Design review of the part built by this model. Coordinates are the model's own, in mm. A direction names the side the tool comes from. Give positions to 0.01 mm unless a question says otherwise; leave off trailing zeros. Order: outer loops, then holes, each group sorted by start corner. A loop starts at its lowest first (then second) coordinate and runs counter-clockwise, first axis right, second up. Notation, with made-up numbers: (18, 7.25) -> (42, 7.25) arc R16 cw to (42, 14.25) -> close; hole circle Ø1 at (22, -6). An arc over 180 degrees is marked (long way). Return JSON: item names as keys, results as strings.
```python
from build123d import *
from build123d.topology import SkipClean

# Parameters (mm, degrees)
SKETCH1_R                     = 27.5
BOSS_EXTRUDE1_DEPTH           = 30
SKETCH4_R                     = 15
BOSS_EXTRUDE3_DEPTH           = 230
BOSS_EXTRUDE3_TAPER           = 1
BOSS_EXTRUDE3_OTHER_WAY_DEPTH = 230
SKETCH2_R                     = 25
CUT_EXTRUDE4_DEPTH            = 20
SKETCH10_R                    = 65.934883456
BOSS_EXTRUDE7_DEPTH           = 5
SKETCH11_R                    = 69.949548389
BOSS_EXTRUDE8_DEPTH           = 5


# Read off the part's stored shape, not the designer's step: Boss-Extrude4, Boss-Extrude5
with BuildPart() as part:
    # Sketch1 → Boss-Extrude1 (new body)
    with BuildSketch(Plane(origin=(0, 0, 0), x_dir=(1, 0, 0), z_dir=(0, 1, 0))):
        with Locations(Location((0, 0, 0), (0, 0, 270))):
            Circle(SKETCH1_R)
    extrude(amount=BOSS_EXTRUDE1_DEPTH)

    # Sketch4 → Boss-Extrude3 (add)
    with BuildSketch(Plane(origin=(0, 0, 0), x_dir=(0, 0, -1), z_dir=(1, 0, 0))):
        with Locations((0, 15)):
            Circle(SKETCH4_R)
    extrude(amount=BOSS_EXTRUDE3_DEPTH, taper=BOSS_EXTRUDE3_TAPER)

    # Sketch4 → Boss-Extrude3 other way (add)
    with SkipClean():  # the faces are left unmerged after this step: merging them gives an invalid solid
        with BuildSketch(Plane(origin=(0, 0, 0), x_dir=(0, 0, -1), z_dir=(1, 0, 0))):
            with Locations((0, 15)):
                Circle(SKETCH4_R)
        extrude(amount=-BOSS_EXTRUDE3_OTHER_WAY_DEPTH)

    # Sketch2 → Cut-Extrude4 (cut)
    with SkipClean():  # the faces are left unmerged after this step: merging them gives an invalid solid
        with BuildSketch(Plane.XZ):
            with Locations(Location((0, 0, 0), (0, 0, 270))):
                Circle(SKETCH2_R)
        extrude(amount=-CUT_EXTRUDE4_DEPTH, mode=Mode.SUBTRACT)

    # Boss-Extrude4 outline → Boss-Extrude4 (revolve)
    with SkipClean():  # the faces are left unmerged after this step: merging them gives an invalid solid
        with BuildSketch(Plane(origin=(0, 15, 0), x_dir=(0, 1, 0), z_dir=(0, 0, -1))):
            Polygon((0, 230), (10.985335067, 230), (65.934883456, 250), (0, 250), align=None)
        revolve(axis=Axis((0, 15, 0), (1, 0, 0)))

    # Boss-Extrude5 outline → Boss-Extrude5 (revolve)
    with SkipClean():  # the faces are left unmerged after this step: merging them gives an invalid solid
        with BuildSketch(Plane(origin=(0, 15, 0), x_dir=(0, 1, 0), z_dir=(0, 0, -1))):
            Polygon((69.949548389, -250), (15, -230), (0, -230), (0, -250), align=None)
        revolve(axis=Axis((0, 15, 0), (1, 0, 0)))

    # Sketch10 → Boss-Extrude7 (add)
    with SkipClean():  # the faces are left unmerged after this step: merging them gives an invalid solid
        with BuildSketch(Plane(origin=(250, 0, 0), x_dir=(0, 0, -1), z_dir=(1, 0, 0))):
            with Locations((0, 15)):
                Circle(SKETCH10_R)
        extrude(amount=BOSS_EXTRUDE7_DEPTH)

    # Sketch11 → Boss-Extrude8 (add)
    with SkipClean():  # the faces are left unmerged after this step: merging them gives an invalid solid
        with BuildSketch(Plane.ZY.offset(250)):
            with Locations((0, 15)):
                Circle(SKETCH11_R)
        extrude(amount=BOSS_EXTRUDE8_DEPTH)

    # Sketch12 → Cut-Revolve3 (revolve, cut)
    with SkipClean():  # the faces are left unmerged after this step: merging them gives an invalid solid
        with BuildSketch(Plane(origin=(0, 15, 0), x_dir=(1, 0, 0), z_dir=(0, 1, 0)), mode=Mode.PRIVATE) as cut_revolve3_sk:
            with BuildLine():
                Line((-234.698463104, 13.289899283), (-253.501037691, 64.949548389))
                Line((-253.501037691, 64.949548389), (-255, 64.949548389))
                Line((-255, 64.949548389), (-255, 0))
                Line((-255, 0), (-234.698463104, 0))
                ThreePointArc((-234.698463104, 0), (-233.526779197, 6.644949642), (-234.698463104, 13.289899283))
            make_face()
        revolve(cut_revolve3_sk.sketch.rotate(Axis((373.268217057, 15, 0), (-1, 0, 0)), 270), axis=Axis((373.268217057, 15, 0), (-1, 0, 0)), mode=Mode.SUBTRACT)

    # Sketch14 → Cut-Revolve4 (revolve, cut)
    with SkipClean():  # the faces are left unmerged after this step: merging them gives an invalid solid
        with BuildSketch(Plane(origin=(0, 15, 0), x_dir=(1, 0, 0), z_dir=(0, 1, 0)), mode=Mode.PRIVATE) as cut_revolve4_sk:
            with BuildLine():
                Line((255, 60.934883456), (253.501037691, 60.934883456))
                Line((253.501037691, 60.934883456), (234.698463104, 9.27523435))
                ThreePointArc((234.698463104, 9.27523435), (233.88072607, 4.637617175), (234.698463104, 0))
                Line((234.698463104, 0), (255, 0))
                Line((255, 0), (255, 60.934883456))
            make_face()
        revolve(cut_revolve4_sk.sketch.rotate(Axis((84.599815478, 15, 0), (1, 0, 0)), 90), axis=Axis((84.599815478, 15, 0), (1, 0, 0)), mode=Mode.SUBTRACT)


solid = part.part
```
Item 1: Add section B-B (x = 203). Give the boundary of the cut face in (y, z).
Result set:
{"outline": "circle Ø22.91 at (15, 0)"}
Item 2: For pin 1 (12 mm diameter, centred on y = 32, z = -6, fed in from +X); pin 2 (1 mm diameter, centred on y = 28, z = -14.5, fed in from +X); pin 3 (3 mm diameter, centred on y = 67.5, z = 7.5, fed in from +X), all flat-tipped, find the tip position at first contact; note any pin that passes through.
Result set:
{"pin 1": "stops at x = 240.07", "pin 2": "stops at x = 238.59", "pin 3": "stops at x = 251.17"}
Item 3: Wall thickness on L1, parallel to Z at x = 0, y = 5.25; L2, parallel to X at y = 21.5, z = -16.5; L3, parallel to X at y = 3, z = 15.5: over which ranges is each line inside the solid? List them lowest first. Write a range as [from, to].
Result set:
{"L1": "z = [-27.5, -25], [25, 27.5]", "L2": "x = [-236.32, -231], [-22, 22], [232.46, 237.78]", "L3": "x = [-237, -231.68], [-22.72, -19.62], [19.62, 22.72], [233.14, 238.46]"}
Item 4: Mouldability with a two-part tool opening along Y and no side actions: class faces 1 (the face through (-22.3, 0, 12.1)), 2 (the face through (-125.076, 0.357, 3.252)), 3 (the face through (235.61, 5.65, -7.17)), 4 (the face through (-254.261, -49.887, -2.856)) as released by +Y, released by -Y, zero draft, split by the parting line, or undercut.
Result set:
{"face 1": "released by -Y", "face 2": "split by the parting line", "face 3": "undercut", "face 4": "undercut"}
Item 5: Add section A-A (x = -122.5). Give the boundary of the cut face in (y, z).
Result set:
{"outline": "circle Ø30 at (15, 0)"}
Item 6: Machinability: for faces 5 (the face through (-230.97, 31.32, -6.77)), 6 (the face through (254.24, -45.876, 2.679)), 7 (the face through (7.509, 9.86, -23.846)), 8 (the face through (0, 30, 0)), which of the approach directions +Z, -Z, +X, -X, +Y, -Y give a long, thin tool a straight path to every point of the face, cutting with its end or side? Answer none if there is none.
Result set:
{"face 5": "none", "face 6": "+X", "face 7": "-Y", "face 8": "+Z, -Z, +Y"}
